Can you work these out from the model? Positions are in its coordinate system, mm. Face numbers are marked on the shaded views. A direction names the side the tool comes from. Round coordinates to 2 decimals unless told otherwise and drop trailing zeros. Loops run counter-clockwise (first coordinate to the right, second up) from the corner with the lowest first, then second, coordinate; pieces in that order, holes last. Notation, with made-up numbers: M 45,-30.5 L 90,-30.5 A32 ccw 90,2.5 Z; hole C 83,-23 d8. An arc over 180 degrees is marked long. Use a Markdown table: item, result. Add a question column.
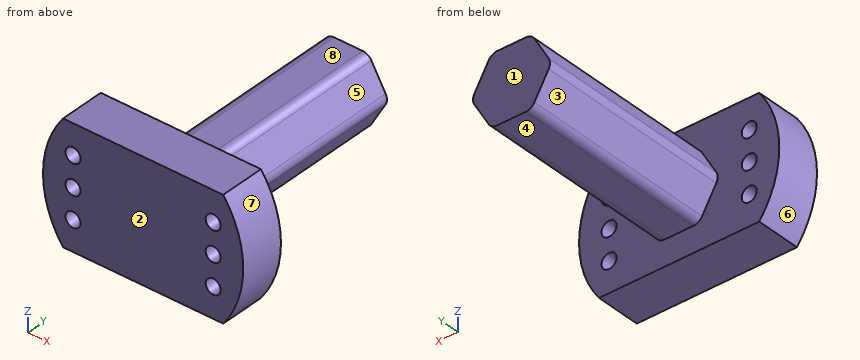
```python
from build123d import *

# Parameters (mm, degrees)
SKETCH_1_R      = 0.75
EXTRUDE_1_DEPTH = 4.5
EXTRUDE_2_DEPTH = 20
FILLET_1_R      = 1


with BuildPart() as part:
    # Эскиз1 → Бобышка-Вытянуть1 (new body)
    with BuildSketch(Plane(origin=(0, 0, 0), x_dir=(1, 0, 0), z_dir=(0, 1, 0))):
        with BuildLine():
            Line((-8, 6), (8, 6))
            ThreePointArc((8, 6), (10, 0), (8, -6))
            Line((8, -6), (-8, -6))
            ThreePointArc((-8, -6), (-10, 0), (-8, 6))
        make_face()
        with Locations(Location((-7, 3, 0), (0, 0, 270))):
            Circle(SKETCH_1_R, mode=Mode.SUBTRACT)
        with Locations(Location((-7, 0, 0), (0, 0, 270))):
            Circle(SKETCH_1_R, mode=Mode.SUBTRACT)
        with Locations(Location((-7, -3, 0), (0, 0, 270))):
            Circle(SKETCH_1_R, mode=Mode.SUBTRACT)
        with Locations(Location((7, -3, 0), (0, 0, 90))):
            Circle(SKETCH_1_R, mode=Mode.SUBTRACT)
        with Locations(Location((7, 0, 0), (0, 0, 90))):
            Circle(SKETCH_1_R, mode=Mode.SUBTRACT)
        with Locations(Location((7, 3, 0), (0, 0, 90))):
            Circle(SKETCH_1_R, mode=Mode.SUBTRACT)
    extrude(amount=EXTRUDE_1_DEPTH)

    # Эскиз2 → Бобышка-Вытянуть2 (add)
    with BuildSketch(Plane(origin=(0, 4.5, 0), x_dir=(1, 0, 0), z_dir=(0, 1, 0))):
        Polygon((2, 3.464101615), (-2, 3.464101615), (-4, 0), (-2, -3.464101615), (2, -3.464101615), (4, 0), align=None)
    extrude(amount=EXTRUDE_2_DEPTH)

    # Скругление1
    fillet_1_edges = [part.edges().sort_by_distance(p)[0] for p in [
        (4, 14.5, 0),
        (2, 14.5, -3.464101615),
        (-2, 14.5, -3.464101615),
        (-4, 14.5, 0),
        (-2, 14.5, 3.464101615),
        (2, 14.5, 3.464101615),
    ]]
    fillet(fillet_1_edges, radius=FILLET_1_R)


solid = part.part
```
(1) Thinking about a two-plate mould opening in Y: for the marked faces 1, 2 and 3, which applies, released by +Y, released by -Y, zero draft, split by the parting line, or undercut?
(2) Suppose I cut it at D-D on x = 2.75. List the corners of the cut face in (y, z) for me.
(3) If I drill on probe 1 along Z at (x, y) = (7, 1.35); probe 2 along X at (y, z) = (1.15, -3); probe 3 along X at (y, z) = (2.55, 0), over which ranges is the centre line in solid material (lowest first)? Write a range as [from, to].
(4) I'm going to push flat-ended pins straight in: pin 1 (0.9 mm diameter, centred on x = 7, z = 0, fed in from -Y); pin 2 (6 mm diameter, centred on y = 14, z = 2.5, fed in from +X); pin 3 (4 mm diameter, centred on x = -5.5, z = -1, fed in from +Y); pin 4 (0.9 mm diameter, centred on x = 0, y = 14, fed in from -Z). Where does each tip first touch, or does it pass through?
(5) Suppose I cut it at A-A on x = 7. List the corners of the cut face in (y, z) for me, and give its area (4 significant figures).
(6) On a 3-axis mill with a long thin cutter (end or side, diameter ignored), from which of +Z, -Z, +X, -X, +Y, -Y can I reach the whole of each face in a straight line? I mean the marked faces 4, 5, 6, 7 and 8. Say none if no direction works.
(7) Suppose I cut it at C-C on y = 19. List the corners of the cut face in (x, z) for me.
(8) Suppose I cut it at B-B on z = 0. List the corners of the cut face in (x, y) for me.
Results below:
| question | item | result |
|---|---|---|
| 1 | face 1 | released by +Y |
| 1 | face 2 | released by -Y |
| 1 | face 3 | zero draft |
| 2 | outline | M 0,-6 L 4.5,-6 L 4.5,-2.17 L 24.5,-2.17 L 24.5,2.17 L 4.5,2.17 L 4.5,6 L 0,6 Z |
| 3 | probe 1 | z = [-6, -3.75], [-2.25, -0.75], [0.75, 2.25], [3.75, 6] |
| 3 | probe 2 | x = [-9.54, -7.75], [-6.25, 6.25], [7.75, 9.54] |
| 3 | probe 3 | x = [-10, -7.75], [-6.25, 6.25], [7.75, 10] |
| 4 | pin 1 | passes through |
| 4 | pin 2 | stops at x = 3.85 |
| 4 | pin 3 | stops at y = 24.5 |
| 4 | pin 4 | stops at z = -3.46 |
| 5 | outline | M 0,-6 L 4.5,-6 L 4.5,-3.75 L 0,-3.75 Z; M 0,-2.25 L 4.5,-2.25 L 4.5,-0.75 L 0,-0.75 Z; M 0,0.75 L 4.5,0.75 L 4.5,2.25 L 0,2.25 Z; M 0,3.75 L 4.5,3.75 L 4.5,6 L 0,6 Z |
| 5 | area | 33.75 mm² |
| 6 | face 4 | -Z, +X, -X, +Y |
| 6 | face 5 | +Z, +X, +Y |
| 6 | face 6 | -X, +Y, -Y |
| 6 | face 7 | +X, +Y, -Y |
| 6 | face 8 | +Z, +X, -X, +Y |
| 7 | outline | M -3.71,-0.5 L -2.29,-2.96 A1 ccw -1.42,-3.46 L 1.42,-3.46 A1 ccw 2.29,-2.96 L 3.71,-0.5 A1 ccw 3.71,0.5 L 2.29,2.96 A1 ccw 1.42,3.46 L -1.42,3.46 A1 ccw -2.29,2.96 L -3.71,0.5 A1 ccw Z |
| 8 | outline | M -10,0 L -7.75,0 L -7.75,4.5 L -10,4.5 Z; M -6.25,0 L 6.25,0 L 6.25,4.5 L 3.85,4.5 L 3.85,24.5 L -3.85,24.5 L -3.85,4.5 L -6.25,4.5 Z; M 7.75,0 L 10,0 L 10,4.5 L 7.75,4.5 Z |
